from build123d import *

# Parameters (mm, degrees)
SKETCH_W        = 85
SKETCH_H        = 65
PAD_DEPTH       = 22
SKETCH001_W     = 80.5
SKETCH001_H     = 60.5
POCKET_DEPTH    = 20
SKETCH002_W     = 83.4
SKETCH002_H     = 63.4
POCKET001_DEPTH = 2
SKETCH003_R     = 1.25
PAD001_DEPTH    = 18
SKETCH004_R     = 2.5
SKETCH004_W     = 25
SKETCH004_H     = 14
POCKET002_DEPTH = 5
SKETCH005_R     = 2.5
SKETCH005_R_2   = 1
PAD002_DEPTH    = 3.5
SKETCH006_W     = 27.4
SKETCH006_H     = 16.4
SKETCH006_W_2   = 25
SKETCH006_H_2   = 14
PAD003_DEPTH    = 1.5
CHAMFER_SIZE2   = 1.5
CHAMFER_SIZE    = 2
CHAMFER001_SIZE = 1.5
SKETCH007_R     = 4
PAD004_DEPTH    = 12
SKETCH008_W     = 10
SKETCH008_H     = 10
POCKET003_DEPTH = 5
POCKET004_DEPTH = 5
SKETCH010_W     = 8
SKETCH010_H     = 9
POCKET005_DEPTH = 5


with BuildPart() as part:
    # Sketch → Pad (new body)
    with BuildSketch(Plane.XY):
        with Locations((42.5, 32.5)):
            Rectangle(SKETCH_W, SKETCH_H)
    extrude(amount=PAD_DEPTH)

    # Sketch001 (on Face6 of Pad) → Pocket (cut)
    with BuildSketch(Plane.XY.offset(22)):
        with Locations((42.5, 32.5)):
            Rectangle(SKETCH001_W, SKETCH001_H)
    extrude(amount=-POCKET_DEPTH, mode=Mode.SUBTRACT)

    # Sketch002 (on Face5 of Pocket) → Pocket001 (cut)
    with BuildSketch(Plane.XY.offset(22)):
        with Locations((42.5, 32.5)):
            Rectangle(SKETCH002_W, SKETCH002_H)
    extrude(amount=-POCKET001_DEPTH, mode=Mode.SUBTRACT)

    # Sketch003 (on Face16 of Pocket001) → Pad001 (join)
    with BuildSketch(Plane.XY.offset(2)):
        with BuildLine():
            Line((2.25, 2.25), (8.25, 2.25))
            Line((8.25, 5), (8.25, 2.25))
            ThreePointArc((8.25, 5), (7.298097, 7.298097), (5, 8.25))
            Line((5, 8.25), (2.25, 8.25))
            Line((2.25, 8.25), (2.25, 2.25))
        make_face()
        with Locations((5, 5)):
            Circle(SKETCH003_R, mode=Mode.SUBTRACT)
        with BuildLine():
            Line((82.75, 2.25), (76.75, 2.25))
            Line((76.75, 5), (76.75, 2.25))
            ThreePointArc((80, 8.25), (77.701903, 7.298097), (76.75, 5))
            Line((80, 8.25), (82.75, 8.25))
            Line((82.75, 8.25), (82.75, 2.25))
        make_face()
        with Locations((80, 5)):
            Circle(SKETCH003_R, mode=Mode.SUBTRACT)
        with BuildLine():
            Line((2.25, 62.75), (8.25, 62.75))
            Line((8.25, 62.75), (8.25, 60))
            ThreePointArc((5, 56.75), (7.298097, 57.701903), (8.25, 60))
            Line((5, 56.75), (2.25, 56.75))
            Line((2.25, 56.75), (2.25, 62.75))
        make_face()
        with Locations((5, 60)):
            Circle(SKETCH003_R, mode=Mode.SUBTRACT)
        with BuildLine():
            Line((82.75, 62.75), (76.75, 62.75))
            Line((76.75, 62.75), (76.75, 60))
            ThreePointArc((76.75, 60), (77.701903, 57.701903), (80, 56.75))
            Line((80, 56.75), (82.75, 56.75))
            Line((82.75, 62.75), (82.75, 56.75))
        make_face()
        with Locations((80, 60)):
            Circle(SKETCH003_R, mode=Mode.SUBTRACT)
    extrude(amount=PAD001_DEPTH)

    # Sketch004 (on Face4 of Pad001) → Pocket002 (cut)
    with BuildSketch(Plane(origin=(0, 0, 0), x_dir=(1, 0, 0), z_dir=(0, 0, -1))):
        with Locations((73, -17)):
            Circle(SKETCH004_R)
        with Locations((60.3, -17)):
            Circle(SKETCH004_R)
        with Locations((47.6, -17)):
            Circle(SKETCH004_R)
        with Locations((25.5, -17)):
            Rectangle(SKETCH004_W, SKETCH004_H)
    extrude(amount=-POCKET002_DEPTH, mode=Mode.SUBTRACT)

    # Sketch005 (on Face18 of Pocket002) → Pad002 (join)
    with BuildSketch(Plane.XY.offset(2)):
        with Locations((15.25, 6.5)):
            Circle(SKETCH005_R)
        with Locations((15.25, 6.5)):
            Circle(SKETCH005_R_2, mode=Mode.SUBTRACT)
        with Locations((35.75, 6.5)):
            Circle(SKETCH005_R)
        with Locations((35.75, 6.5)):
            Circle(SKETCH005_R_2, mode=Mode.SUBTRACT)
        with Locations((35.75, 29.5)):
            Circle(SKETCH005_R)
        with Locations((35.75, 29.5)):
            Circle(SKETCH005_R_2, mode=Mode.SUBTRACT)
        with Locations((15.25, 29.5)):
            Circle(SKETCH005_R)
        with Locations((15.25, 29.5)):
            Circle(SKETCH005_R_2, mode=Mode.SUBTRACT)
    extrude(amount=PAD002_DEPTH)

    # Sketch006 (on Face18 of Pad002) → Pad003 (join)
    with BuildSketch(Plane.XY.offset(2)):
        with Locations((25.5, 17)):
            Rectangle(SKETCH006_W, SKETCH006_H)
        with Locations((25.5, 17)):
            Rectangle(SKETCH006_W_2, SKETCH006_H_2, mode=Mode.SUBTRACT)
    extrude(amount=PAD003_DEPTH)

    # Chamfer
    chamfer_edges = [part.edges().sort_by_distance(p)[0] for p in [
        (25.5, 10, 0),
        (13, 17, 0),
        (25.5, 24, 0),
        (38, 17, 0),
    ]]
    chamfer_side = part.faces().sort_by_distance((43.458054, 33.73884, 0))[0]
    chamfer(chamfer_edges, length=CHAMFER_SIZE, length2=CHAMFER_SIZE2, reference=chamfer_side)

    # Chamfer001
    chamfer001_edges = [part.edges().sort_by_distance(p)[0] for p in [
        (0, 32.5, 0),
        (42.5, 65, 0),
        (85, 32.5, 0),
        (42.5, 0, 0),
    ]]
    chamfer(chamfer001_edges, length=CHAMFER001_SIZE)

    # Sketch007 (on Face21 of Chamfer001) → Pad004 (join)
    with BuildSketch(Plane.XY.offset(2)):
        with BuildLine():
            ThreePointArc((68.390228, 14), (78.5, 17), (68.390228, 20))
            ThreePointArc((64.909772, 20), (66.65, 19.443687), (68.390228, 20))
            ThreePointArc((64.909772, 20), (60.3, 22.5), (55.690228, 20))
            ThreePointArc((52.209772, 20), (53.95, 19.443687), (55.690228, 20))
            ThreePointArc((52.209772, 20), (42.1, 17), (52.209772, 14))
            ThreePointArc((55.690228, 14), (53.95, 14.556313), (52.209772, 14))
            ThreePointArc((55.690228, 14), (60.3, 11.5), (64.909772, 14))
            ThreePointArc((68.390228, 14), (66.65, 14.556313), (64.909772, 14))
        make_face()
        with Locations((47.6, 17)):
            Circle(SKETCH007_R, mode=Mode.SUBTRACT)
        with Locations((60.3, 17)):
            Circle(SKETCH007_R, mode=Mode.SUBTRACT)
        with Locations((73, 17)):
            Circle(SKETCH007_R, mode=Mode.SUBTRACT)
    extrude(amount=PAD004_DEPTH)

    # Sketch008 (on Face14 of Pad004) → Pocket003 (cut)
    with BuildSketch(Plane(origin=(0, 65, 0), x_dir=(-1, 0, 0), z_dir=(0, 1, 0))):
        with Locations((-62, 17)):
            Rectangle(SKETCH008_W, SKETCH008_H)
    extrude(amount=-POCKET003_DEPTH, mode=Mode.SUBTRACT)

    # Sketch009 (on Face14 of Pocket003) → Pocket004 (cut)
    with BuildSketch(Plane(origin=(0, 65, 0), x_dir=(-1, 0, 0), z_dir=(0, 1, 0))):
        with BuildLine():
            ThreePointArc((-19, 17.5), (-14, 12.5), (-9, 17.5))
            Line((-9, 22), (-9, 17.5))
            Line((-19, 22), (-9, 22))
            Line((-19, 17.5), (-19, 22))
        make_face()
        with BuildLine():
            ThreePointArc((-33, 17.5), (-28, 12.5), (-23, 17.5))
            Line((-23, 22), (-23, 17.5))
            Line((-33, 22), (-23, 22))
            Line((-33, 17.5), (-33, 22))
        make_face()
    extrude(amount=-POCKET004_DEPTH, mode=Mode.SUBTRACT)

    # Sketch010 (on Face15 of Pocket004) → Pocket005 (cut)
    with BuildSketch(Plane.XZ):
        with Locations((65, 17.5)):
            Rectangle(SKETCH010_W, SKETCH010_H)
    extrude(amount=-POCKET005_DEPTH, mode=Mode.SUBTRACT)


solid = part.part
Part model, mm, in its own coordinate system. A direction names the side the tool comes from. Give positions to 0.01 mm unless a question says otherwise; leave off trailing zeros. Order: outer loops, then holes, each group sorted by start corner. A loop starts at its lowest first (then second) coordinate and runs counter-clockwise, first axis right, second up. Notation, with made-up numbers: (42.25, 47.5) -> (78.25, 47.5) arc R34 ccw to (78.25, 79.5) -> close; hole circle Ø6 at (53.25, 13.5). An arc over 180 degrees is marked (long way). Use one line per item in the form item = value.
(1) Flat gauge pins, fed straight in: P1, Ø2, axis at x = 5, y = 60, coming from the +Z side; P2, Ø6, axis at x = 47.5, z = 14.5, coming from the -Y side; P3, Ø2.5, axis at x = 15.25, y = 6.5, coming from the +Z side; P4, Ø1.8, axis at x = 66, y = 1.5, coming from the +Z side. Where does each tip first touch, or does it go through?
Solution:
P1 = 2
P2 = 0
P3 = 5.5
P4 = 13
(2) Tool access for faces 3 (the face through (23, 64, 19)), 4 (the face through (25.3, 24.99, 0.76)), 5 (the face through (42.104, 17.197, 7.916)): list every direction of +Z, -Z, +X, -X, +Y, -Y with a clear straight run to the whole face (end or side of a thin tool).
Solution:
face_3 = +Z, +Y
face_4 = -Z
face_5 = +Z
(3) Pull direction Y, two halves, no side cores. Call faces 1 (the face through (28.1, 63.9, 12.5)), 2 (the face through (48, 14, 2)): +Y half, -Y half, draft (parallel to the pull), parting line (faces both ways), or undercut.
Solution:
face_1 = draft
face_2 = undercut
(4) Saw through at B-B (z = 9.5). Count the separate pieces of the cut face and the enclosed holes in it, then the cut area to 3 significant figures.
Solution:
separate_pieces = 2
enclosed_holes = 8
area = 926 mm²
(5) Drill centre lines: line 1 (Y direction, x = 60.3, z = 5.5); line 2 (Y direction, x = 35.75, z = 3.6); line 3 (Y direction, x = 10.5, z = 5.5). Where is each one in solid material? Low to high. Write a range as from..to.
Solution:
line_1 = 0..2.25, 11.5..13, 21..22.5, 62.75..65
line_2 = 0..2.25, 4..5.5, 7.5..9, 27..28.5, 30.5..32, 62.75..65
line_3 = 0..2.25, 62.75..65
(6) Saw through at C-C (y = 34). Write the cut outline in (x, z), then the cut area to 3 significant figures.
Solution:
outline = (0, 1.5) -> (1.5, 0) -> (83.5, 0) -> (85, 1.5) -> (85, 22) -> (84.2, 22) -> (84.2, 20) -> (82.75, 20) -> (82.75, 2) -> (2.25, 2) -> (2.25, 20) -> (0.8, 20) -> (0.8, 22) -> (0, 22) -> close
area = 252 mm²
(7) Saw through at A-A (x = 73). Write the cut outline in (y, z).
Solution:
outline = (0, 1.5) -> (1.5, 0) -> (14.5, 0) -> (14.5, 2) -> (13, 2) -> (13, 14) -> (11.5, 14) -> (11.5, 2) -> (2.25, 2) -> (2.25, 20) -> (0.8, 20) -> (0.8, 22) -> (0, 22) -> close; (19.5, 0) -> (63.5, 0) -> (65, 1.5) -> (65, 22) -> (64.2, 22) -> (64.2, 20) -> (62.75, 20) -> (62.75, 2) -> (22.5, 2) -> (22.5, 14) -> (21, 14) -> (21, 2) -> (19.5, 2) -> close
